Input: part model. Units: mm. Frame: model coordinates. Coordinates: 2 decimals unless noted, no trailing zeros. Order: outer loops, then holes, each group sorted by start corner. A loop starts at its lowest first (then second) coordinate and runs counter-clockwise, first axis right, second up. Notation, with made-up numbers: (79.5, -26.5) -> (132.5, -26.5) arc R12 cw to (132.5, -3.5) -> close; hole circle Ø6 at (62, 19). An arc over 180 degrees is marked (long way). Write each question's results on one line, items separated by ' | '.
```python
from build123d import *

# Parameters (mm, degrees)
F0_R       = 10
F1_DEPTH   = 25
F2_DEPTH   = 25
F3_R       = 5
F1_FACE1_R = 10
F5_T       = -1.5


with BuildPart() as f1:
    # F0 (on Front) → F1 (new body)
    with BuildSketch(Plane.XZ):
        Circle(F0_R)
    extrude(amount=F1_DEPTH)

    # F2 (add): a face of the model
    f2_faces = [f1.faces().sort_by_distance(p)[0] for p in [
        (0, 0, 0),
    ]]
    extrude(f2_faces, amount=F2_DEPTH)

    # F3 (on face) → F4 section 0
    with BuildSketch(Plane(origin=(0, 25, 0), x_dir=(-1, 0, 0), z_dir=(0, 1, 0))):
        Circle(F3_R)
    # F1_face1 (on face) → F4 section 1
    with BuildSketch(Plane.XZ.offset(25)):
        Circle(F1_FACE1_R)
    loft(mode=Mode.INTERSECT)

    # F5
    f5_openings = [f1.faces().sort_by_distance(p)[0] for p in [
        (0, -25, 0),
        (0, 25, 0),
    ]]
    offset(amount=F5_T, openings=f5_openings, kind=Kind.INTERSECTION)


solid = f1.part
```
(1) Cut plane A-A, the plane x = 0. Return loops of the section in (y, z), plus the area to 3 significant figures.
Return value:
outline: (-25, -10) -> (25, -5) -> (25, -3.49) -> (-25, -8.49) -> close; (-25, 8.49) -> (25, 3.49) -> (25, 5) -> (-25, 10) -> close | area: 151 mm2
(2) Mould query, pull axis X, two halves, no side actions, for faces 1 (the face through (-4.5, -25, -7.4)), 2 (the face through (4.78, -0.35, -3.67)), 3 (the face through (5.98, -0.35, -4.585)). Classes: +X half, -X half, draft (parallel to the pull), parting line (faces both ways), or undercut.
Return value:
face 1: draft | face 2: undercut | face 3: parting line
(3) Line query: line 1 along Z through (x, y) = (-4.25, -9.5); line 2 along Z through (x, y) = (5, 3.5); line 3 along X through (y, z) = (21, 2.25). Output: solid intervals per line, ascending. Write a range as from..to.
Return value:
line 1: -7.3..-5.49, 5.49..7.3 | line 2: -5.11..-2.61, 2.61..5.11 | line 3: -4.91..-3.18, 3.18..4.91
(4) Cut plane C-C, the plane y = 12. Return loops of the section in (x, z), plus the area to 3 significant figures.
Return value:
outline: circle Ø12.6 at (0, 0); hole circle Ø9.59 at (0, 0) | area: 52.5 mm2
(5) Cut plane B-B, the plane y = -14.5. Return loops of the section in (x, z).
Return value:
outline: circle Ø17.9 at (0, 0); hole circle Ø14.89 at (0, 0)
(6) Pin query (flat end, axial travel): P1, Ø12, axis at y = -17.5, z = 3, coming from the -X side; P2, Ø1.5, axis at y = -11, z = -5, coming from the +X side; P3, Ø1, axis at x = -3.5, y = -4.5, coming from the -Z side. Return the tip coordinate at first contact, or that it passes through.
Return value:
P1: x = -9.78 | P2: x = 7.49 | P3: z = -7.37
